from build123d import *

# Parameters (mm, degrees)
EXTRUDE1_DEPTH              = 19.05
F_5_16_18_TAPPED_HOLE1_D    = 6.5278
F_3_8_24_TAPPED_HOLE1_D     = 8.4328
F_3_8_24_TAPPED_HOLE1_DEPTH = 12.7
F_3_8_24_TAPPED_HOLE1_TIP   = 2.533468714


with BuildPart() as part:
    # Sketch1 → Extrude1 (new body)
    with BuildSketch(Plane(origin=(0, 0, 0), x_dir=(0, 0, -1), z_dir=(1, 0, 0))):
        Polygon((0, 0), (11.90625, 0), (11.90625, 50.8), (-7.14375, 50.8), (-7.14375, 19.84375), (0, 19.84375), align=None)
    extrude(amount=EXTRUDE1_DEPTH)

    # 5/16-18 Tapped Hole1 (through all)
    with Locations(Plane.XY.offset(7.14375)):
        with Locations((9.525, 31.75)):
            Hole(F_5_16_18_TAPPED_HOLE1_D / 2)

    # 3/8-24 Tapped Hole1
    with Locations(Plane(origin=(0, 50.8, 0), x_dir=(-1, 0, 0), z_dir=(0, 1, 0))):
        with Locations((-9.525, 0.79375)):
            Hole(F_3_8_24_TAPPED_HOLE1_D / 2, depth=F_3_8_24_TAPPED_HOLE1_DEPTH)
            with Locations((0, 0, -(F_3_8_24_TAPPED_HOLE1_DEPTH + F_3_8_24_TAPPED_HOLE1_TIP / 2))):  # 118° drill point
                Cone(0, F_3_8_24_TAPPED_HOLE1_D / 2, F_3_8_24_TAPPED_HOLE1_TIP, mode=Mode.SUBTRACT)


solid = part.part
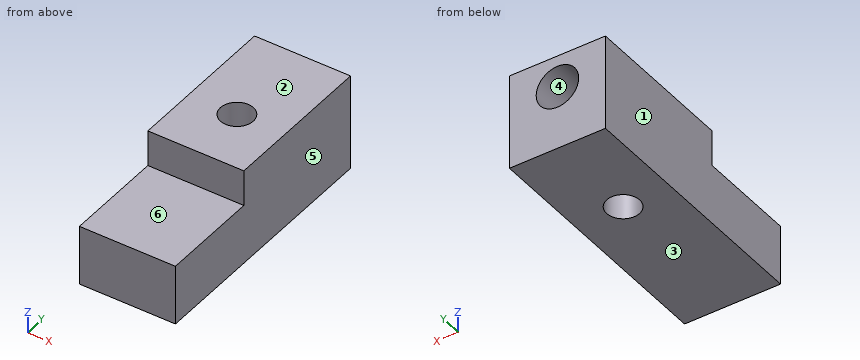
Geometry: final body of the model. Coordinates: model frame, mm. Face numbers are marked on the shaded views. A direction names the side the tool comes from. Coordinates: 2 decimals unless noted, no trailing zeros. Write each loop counter-clockwise with the first axis right and the second up, starting at its lowest first coordinate (ties: lowest second). Pieces come first, ordered by that corner, then holes. Notation, with made-up numbers: (86, -34) - (96, -34) arc R22 cw to (96, 5) - close; hole circle Ø1 at (-4.75, 38). An arc over 180 degrees is marked (long way). Return JSON: item names as keys, results as strings.
Item 1: Reachability of the marked faces 5 and 6 from +Z, -Z, +X, -X, +Y, -Y: full face, straight path, thin tool, end or side. Return the list, or none.
Completed:
{"face 5": "+Z, -Z, +X, +Y, -Y", "face 6": "+Z, +X, -X, -Y"}
Item 2: Section query D-D (y = 13.5). Output: boundary loops of the cut face in (x, z).
Completed:
{"outline": "(0, -11.91) - (19.05, -11.91) - (19.05, 0) - (0, 0) - close"}
Item 3: Section query A-A (y = 31.75). Output: boundary loops of the cut face in (x, z), and give its area (3 significant figures).
Completed:
{"outline": "(0, -11.91) - (6.26, -11.91) - (6.26, 7.14) - (0, 7.14) - close; (12.79, -11.91) - (19.05, -11.91) - (19.05, 7.14) - (12.79, 7.14) - close", "area": "239 mm2"}
Item 4: Pull-direction query (Z, two-part tool) for the marked faces 1, 2, 3 and 4; classes: +Z half, -Z half, draft (parallel to the pull), parting line (faces both ways), or undercut.
Completed:
{"face 1": "draft", "face 2": "+Z half", "face 3": "-Z half", "face 4": "undercut"}
Item 5: Section query B-B (z = -4). Output: boundary loops of the cut face in (x, y) (3 decimals), and give its area (3 significant figures).
Completed:
{"outline": "(0, 0) - (19.05, 0) - (19.05, 50.8) - (0, 50.8) - close; hole circle Ø6.528 at (9.525, 31.75)", "area": "934 mm2"}
Item 6: Pin query (flat end, axial travel): pin 1 Ø4 at (x, y) = (9.525, 31.75) entering from +Z; pin 2 Ø5.5 at (x, y) = (11, 11) entering from +Z; pin 3 Ø5 at (x, z) = (9.52, 0.79) entering from +Y; pin 4 Ø3.5 at (x, z) = (7, 5) entering from -Y. Return the tip coordinate at first contact, or that it passes through.
Completed:
{"pin 1": "passes through", "pin 2": "stops at z = 0", "pin 3": "stops at y = 37.07", "pin 4": "stops at y = 19.84"}
Item 7: Section query C-C (x = 15.75). Output: boundary loops of the cut face in (y, z), and give its area (3 significant figures).
Completed:
{"outline": "(0, -11.91) - (50.8, -11.91) - (50.8, 7.14) - (19.84, 7.14) - (19.84, 0) - (0, 0) - close", "area": "826 mm2"}
Item 8: Line query: L1, parallel to X at y = 43, z = 1; L2, parallel to Y at x = 10.5, z = -4; L3, parallel to Y at x = 8.5, z = -6. Output: solid intervals per line, ascending.
Completed:
{"L1": "x = 0 to 5.31, 13.74 to 19.05", "L2": "y = 0 to 28.64, 34.86 to 50.8", "L3": "y = 0 to 28.65, 34.85 to 50.8"}
